Part model, mm, in its own coordinate system. A direction names the side the tool comes from. Give positions to 0.01 mm unless a question says otherwise; leave off trailing zeros. Order: outer loops, then holes, each group sorted by start corner. A loop starts at its lowest first (then second) coordinate and runs counter-clockwise, first axis right, second up.
1. Drop flat-ended pins along their axis: pin 1 Ø0.5 at (x, y) = (16.5, 0.5) entering from +Z; pin 2 Ø0.8 at (x, y) = (17, 1) entering from -Z. Give the stop position or say it passes through.
2. Slice it at B-B on x = 6. List the corners of the cut face in (y, z).
3. Slice it at C-C on z = -7. List the corners of the cut face in (x, y), and give its area (3 significant figures).
4. Slice it at A-A on y = 0.7. Give the number of separate pieces and of enclosed holes in the cut face, and give its area (3 significant figures).
5. Probe line 1 (Z direction, x = -9.51, y = 0.85); line 2 (X direction, y = 0.7, z = 16.75); line 3 (Z direction, x = -12.05, y = 0.85). List the from-to ranges inside material, lowest first.
6. Which spindle directions (+Z, -Z, +X, -X, +Y, -Y) get a long thin tool onto all of the face, cutting with end or side? Do faces 1 (the flat face through (-14.5, 1, 0)), 2 (the flat face through (14.5, 1, 20)), 3 (the flat face through (14.5, 1, -12)), 4 (the flat face through (-10.8, 1, 25)), 5 (the flat face through (-4, 1, 25.4)). Say none if no direction does.
Autodesk Inventor part; units mm, degrees
ref_plane "YZ Plane" through (0, 0, 0) normal (1, 0, 0) x (0, 1, 0)
ref_plane "XZ Plane" through (0, 0, 0) normal (0, 1, 0) x (-1, 0, 0)
ref_plane "XY Plane" through (0, 0, 0) normal (0, 0, 1) x (1, 0, 0)
sketch "Sketch1" plane through (0, 0, 0) normal (0, 1, 0) x (-1, 0, 0)
  line L0 (14.5, -22.6) -> (-14.5, -22.6)
  line L1 (-14.5, -22.6) -> (-14.5, 22.6)
  line L2 (-14.5, 22.6) -> (14.5, 22.6)
  line L3 (14.5, 22.6) -> (14.5, -22.6)
  point P0 (0, 0)
  point P1 (0, -22.6)
  point P2 (14.5, 0)
  dimension "d0" = 29
  dimension "d1" = 45.2
extrude "Extrusion1" add sketch "Sketch1" along normal blind 1.6
sketch "Sketch2" plane through (0, 1.6, 0) normal (0, 1, 0) x (1, 0, 0)
  line L0 (14.5, 22.6) -> (-14.5, 22.6)
  line L1 (-14.5, 22.6) -> (-14.5, -22.6)
  line L2 (-14.5, -22.6) -> (14.5, -22.6)
  line L3 (14.5, -22.6) -> (14.5, 22.6)
  line L4 (14.5, 0.35) -> (17.5, 0.35)
  line L5 (17.5, 0.35) -> (17.5, -15.6)
  line L6 (17.5, -15.6) -> (14.5, -15.6)
  line L7 (14.5, -15.6) -> (14.5, 0.35)
  point P0 (0, 0)
  point P1 (14.5, -7.625)
  point P2 (14.5, 0)
  dimension "d4" = 3
  dimension "d5" = 15.95
  dimension "d6" = 7
extrude "Extrusion2" add sketch "Sketch2" against normal up to surface (1.6 mm away) contours L4 L5 L6 L3
sketch "Sketch3" plane through (0, 1.6, 0) normal (0, 1, 0) x (1, 0, 0)
  line L0 (14.5, 22.6) -> (-14.5, 22.6)
  line L1 (-14.5, 22.6) -> (-14.5, -22.6)
  line L2 (-14.5, -22.6) -> (14.5, -22.6)
  line L3 (14.5, -22.6) -> (14.5, -15.6)
  line L4 (17.5, -15.6) -> (14.5, -15.6)
  line L5 (17.5, 0.35) -> (17.5, -15.6)
  line L6 (14.5, 0.35) -> (17.5, 0.35)
  line L7 (14.5, 0.35) -> (14.5, 22.6)
  line L8 (-10.8, -22.6) -> (3.5, -22.6)
  line L9 (3.5, -22.6) -> (3.5, -25.4)
  line L10 (3.5, -25.4) -> (-10.8, -25.4)
  line L11 (-10.8, -25.4) -> (-10.8, -22.6)
  line L12 (-14.5, -22.6) -> (14.5, -22.6)
  point P0 (0, 0)
  point P1 (-3.65, -22.6)
  point P2 (0, -22.6)
  dimension "d9" = 2.8
  dimension "d10" = 14.3
  dimension "d11" = 3.7
extrude "Extrusion3" add sketch "Sketch3" against normal up to surface (1.6 mm away) contours L2 L9 L10 L11
fillet "Fillet1" radius 1.27 4 edges at (-10.8, 0.8, 22.6) (3.5, 0.8, 22.6) (14.5, 0.8, 15.6) (14.5, 0.8, -0.35)
sketch "Sketch4" plane through (0, 1.6, 0) normal (0, 1, 0) x (1, 0, 0)
  line L0 (14.5, 22.6) -> (-14.5, 22.6)
  line L1 (-14.5, 22.6) -> (-14.5, -22.6)
  line L2 (-14.5, -22.6) -> (-12.07, -22.6)
  arc A0 (-10.8, -23.87) -> (-12.07, -22.6) centre (-12.07, -23.87) ccw
  line L3 (-10.8, -25.4) -> (-10.8, -23.87)
  line L4 (3.5, -25.4) -> (-10.8, -25.4)
  line L5 (3.5, -23.87) -> (3.5, -25.4)
  arc A1 (4.77, -22.6) -> (3.5, -23.87) centre (4.77, -23.87) ccw
  line L6 (4.77, -22.6) -> (14.5, -22.6)
  line L7 (14.5, -22.6) -> (14.5, -16.87)
  arc A2 (15.77, -15.6) -> (14.5, -16.87) centre (15.77, -16.87) ccw
  line L8 (17.5, -15.6) -> (15.77, -15.6)
  line L9 (17.5, 0.35) -> (17.5, -15.6)
  line L10 (15.77, 0.35) -> (17.5, 0.35)
  arc A3 (14.5, 1.62) -> (15.77, 0.35) centre (15.77, 1.62) ccw
  line L11 (14.5, 1.62) -> (14.5, 22.6)
  point P0 (0, 0)
  point P1 (12.15, -20.2)
  point P2 (9.15, -20.2)
  dimension "d15" = 2.35
  dimension "d16" = 2.4
  dimension "d17" = 2.4
  dimension "d18" = 5.35
hole "Hole1" at (12.15, 1.6, 20.2) at (9.15, 1.6, 20.2) direction (0, -1, 0) diameter 0.8 end through all
sketch "Sketch5" plane through (0, 1.6, 0) normal (0, 1, 0) x (1, 0, 0)
  circle A0 centre (12.15, -20.2) radius 0.4
  circle A1 centre (9.15, -20.2) radius 0.4
  line L0 (14.5, 22.6) -> (-14.5, 22.6)
  line L1 (-14.5, 22.6) -> (-14.5, -22.6)
  line L2 (-14.5, -22.6) -> (-12.07, -22.6)
  arc A2 (-10.8, -23.87) -> (-12.07, -22.6) centre (-12.07, -23.87) ccw
  line L3 (-10.8, -25.4) -> (-10.8, -23.87)
  line L4 (3.5, -25.4) -> (-10.8, -25.4)
  line L5 (3.5, -23.87) -> (3.5, -25.4)
  arc A3 (4.77, -22.6) -> (3.5, -23.87) centre (4.77, -23.87) ccw
  line L6 (4.77, -22.6) -> (14.5, -22.6)
  line L7 (14.5, -22.6) -> (14.5, -16.87)
  arc A4 (15.77, -15.6) -> (14.5, -16.87) centre (15.77, -16.87) ccw
  line L8 (17.5, -15.6) -> (15.77, -15.6)
  line L9 (17.5, 0.35) -> (17.5, -15.6)
  line L10 (15.77, 0.35) -> (17.5, 0.35)
  arc A5 (14.5, 1.62) -> (15.77, 0.35) centre (15.77, 1.62) ccw
  line L11 (14.5, 1.62) -> (14.5, 22.6)
  line L12 (-12.05, -19.95) -> (-12.05, -17) construction
  line L13 (-12.05, -19.95) -> (-11.6759, -19.95) construction
  point P0 (0, 0)
  point P1 (-12.05, -18.35)
  point P2 (-12.05, -16.75)
  point P3 (-9.51, -19.95)
  point P4 (-9.51, -18.35)
  point P5 (-9.51, -16.75)
  dimension "d26" = 2.65
  dimension "d27" = 2.45
  dimension "d30" = 1.6
  dimension "d33" = 2.54
hole "Hole2" at (-12.05, 1.6, 19.95) at (-12.05, 1.6, 18.35) at (-12.05, 1.6, 16.75) at (-9.51, 1.6, 19.95) at (-9.51, 1.6, 18.35) at (-9.51, 1.6, 16.75) direction (0, -1, 0) diameter 0.8 end through all
sketch "Sketch6" plane through (0, 1.6, 0) normal (0, 1, 0) x (1, 0, 0)
  circle A0 centre (-9.51, -18.35) radius 0.4
  circle A1 centre (-12.05, -16.75) radius 0.4
  circle A2 centre (-12.05, -19.95) radius 0.4
  circle A3 centre (-12.05, -18.35) radius 0.4
  circle A4 centre (-9.51, -19.95) radius 0.4
  circle A5 centre (-9.51, -16.75) radius 0.4
  circle A6 centre (12.15, -20.2) radius 0.4
  circle A7 centre (9.15, -20.2) radius 0.4
  line L0 (14.5, 22.6) -> (-14.5, 22.6)
  line L1 (-14.5, 22.6) -> (-14.5, -22.6)
  line L2 (-14.5, -22.6) -> (-12.07, -22.6)
  arc A8 (-10.8, -23.87) -> (-12.07, -22.6) centre (-12.07, -23.87) ccw
  line L3 (-10.8, -25.4) -> (-10.8, -23.87)
  line L4 (3.5, -25.4) -> (-10.8, -25.4)
  line L5 (3.5, -23.87) -> (3.5, -25.4)
  arc A9 (4.77, -22.6) -> (3.5, -23.87) centre (4.77, -23.87) ccw
  line L6 (4.77, -22.6) -> (14.5, -22.6)
  line L7 (14.5, -22.6) -> (14.5, -16.87)
  arc A10 (15.77, -15.6) -> (14.5, -16.87) centre (15.77, -16.87) ccw
  line L8 (17.5, -15.6) -> (15.77, -15.6)
  line L9 (17.5, 0.35) -> (17.5, -15.6)
  line L10 (15.77, 0.35) -> (17.5, 0.35)
  arc A11 (14.5, 1.62) -> (15.77, 0.35) centre (15.77, 1.62) ccw
  line L11 (14.5, 1.62) -> (14.5, 22.6)
  point P0 (0, 0)
properties part number "BarePCB"
Data:
1. pin 1: stops at z = 15.6
1. pin 2: stops at z = -0.35
2. outline: (0, -22.6) - (1.6, -22.6) - (1.6, 22.6) - (0, 22.6) - close
3. outline: (-14.5, 0) - (14.5, 0) - (14.5, 1.6) - (-14.5, 1.6) - close
3. area: 46.4 mm2
4. separate pieces: 1
4. enclosed holes: 8
4. area: 1,400 mm2
5. line 1: z = -22.6 to 16.35, 17.15 to 17.95, 18.75 to 19.55, 20.35 to 25.4
5. line 2: x = -14.5 to -12.45, -11.65 to -9.91, -9.11 to 14.51
5. line 3: z = -22.6 to 16.35, 17.15 to 17.95, 18.75 to 19.55, 20.35 to 22.6
6. face 1: +Z, -Z, -X, +Y, -Y
6. face 2: +Z, +X, +Y, -Y
6. face 3: -Z, +X, +Y, -Y
6. face 4: +Z, -X, +Y, -Y
6. face 5: +Z, +X, -X, +Y, -Y
